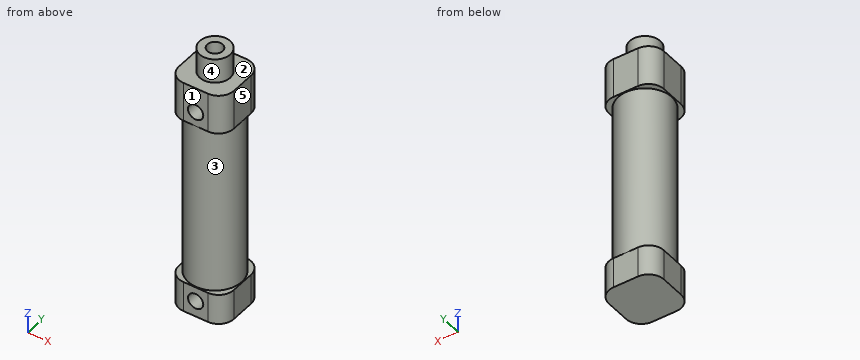
```python
from build123d import *

# Parameters (mm, degrees)
SKETCH_1_W          = 18
SKETCH_1_H          = 18
EXTRUDE_1_DEPTH     = 10
SKETCH_2_R          = 8.75
EXTRUDE_2_DEPTH     = 55.5
SKETCH_3_W          = 18
SKETCH_3_H          = 18
EXTRUDE_3_DEPTH     = 13
SKETCH_4_R          = 5
EXTRUDE_4_DEPTH     = 8
SKETCH_5_R          = 2.5
CUT_EXTRUDE_1_DEPTH = 85.5
FILLET_1_R          = 5
CUT_EXTRUDE_2_REACH = 20
SKETCH_6_R          = 2.5


with BuildPart() as part:
    # 草图1 → 凸台-拉伸1 (new body)
    with BuildSketch(Plane.XY):
        Rectangle(SKETCH_1_W, SKETCH_1_H)
    extrude(amount=EXTRUDE_1_DEPTH)

    # 草图2 → 凸台-拉伸2 (add)
    with BuildSketch(Plane.XY.offset(10)):
        Circle(SKETCH_2_R)
    extrude(amount=EXTRUDE_2_DEPTH)

    # 草图3 → 凸台-拉伸3 (add)
    with BuildSketch(Plane.XY.offset(65.5)):
        Rectangle(SKETCH_3_W, SKETCH_3_H)
    extrude(amount=EXTRUDE_3_DEPTH)

    # 草图4 → 凸台-拉伸4 (add)
    with BuildSketch(Plane.XY.offset(78.5)):
        Circle(SKETCH_4_R)
    extrude(amount=EXTRUDE_4_DEPTH)

    # 草图5 → 切除-拉伸1 (cut)
    with BuildSketch(Plane.XY.offset(86.5)):
        Circle(SKETCH_5_R)
    extrude(amount=-CUT_EXTRUDE_1_DEPTH, mode=Mode.SUBTRACT)

    # 圆角1
    fillet_1_edges = [part.edges().sort_by_distance(p)[0] for p in [
        (9, -9, 72),
        (9, 9, 72),
        (-9, 9, 72),
        (-9, -9, 72),
        (9, -9, 5),
        (-9, -9, 5),
        (-9, 9, 5),
        (9, 9, 5),
    ]]
    fillet(fillet_1_edges, radius=FILLET_1_R)

    # 草图6 → 切除-拉伸2 (cut, up to next)
    with BuildSketch(Plane.XZ.offset(9), mode=Mode.PRIVATE) as cut_extrude_2_sk1:
        with Locations((0, 5.25)):
            Circle(SKETCH_6_R)
    cut_extrude_2_tool1 = extrude(cut_extrude_2_sk1.sketch, amount=-CUT_EXTRUDE_2_REACH, mode=Mode.PRIVATE) & part.part
    add(cut_extrude_2_tool1.solids().sort_by_distance((0, -9, 5.25))[0], mode=Mode.SUBTRACT)
    # 草图6 → 切除-拉伸2 (cut, up to next)
    with BuildSketch(Plane.XZ.offset(9), mode=Mode.PRIVATE) as cut_extrude_2_sk2:
        with Locations((0, 70.25)):
            Circle(SKETCH_6_R)
    cut_extrude_2_tool2 = extrude(cut_extrude_2_sk2.sketch, amount=-CUT_EXTRUDE_2_REACH, mode=Mode.PRIVATE) & part.part
    add(cut_extrude_2_tool2.solids().sort_by_distance((0, -9, 70.25))[0], mode=Mode.SUBTRACT)


solid = part.part
```
Verification items for the finished model (mm, model axes). Face numbers are marked on the shaded views. A direction names the side the tool comes from. Round coordinates to 2 decimals unless told otherwise and drop trailing zeros. Order: outer loops, then holes, each group sorted by start corner. A loop starts at its lowest first (then second) coordinate and runs counter-clockwise, first axis right, second up.
1) Cross-section at C-C, the plane z = 76. Record the cut outline in (x, y), plus the area to 3 significant figures.
Geometry says:
outline: (-9, -4) arc R5 ccw to (-4, -9) - (4, -9) arc R5 ccw to (9, -4) - (9, 4) arc R5 ccw to (4, 9) - (-4, 9) arc R5 ccw to (-9, 4) - close; hole circle Ø5 at (0, 0)
area: 283 mm2
2) Draft check along Z on the marked faces 1, 2 and 3. Enter one of: +Z half, -Z half, draft (parallel to the pull), parting line (faces both ways), or undercut.
Geometry says:
face 1: draft
face 2: +Z half
face 3: undercut
3) Depth check by flat-ended pin: pin 1 (4 mm diameter, centred on x = -5.5, z = 26, fed in from -Y); pin 2 (6 mm diameter, centred on y = -6, z = 42.5, fed in from -X); pin 3 (1 mm diameter, centred on y = 6.5, z = 69.5, fed in from +X). Enter the tip coordinate at first touch or a pass-through.
Geometry says:
pin 1: stops at y = -8.02
pin 2: stops at x = -8.22
pin 3: stops at x = 8.58
4) Cross-section at B-B, the plane x = -7. Record the cut outline in (y, z), plus the area to 3 significant figures.
Geometry says:
outline: (-8, 0) - (8, 0) - (8, 10) - (5.25, 10) - (5.25, 65.5) - (8, 65.5) - (8, 78.5) - (-8, 78.5) - (-8, 65.5) - (-5.25, 65.5) - (-5.25, 10) - (-8, 10) - close
area: 951 mm2
5) Cross-section at D-D, the plane y = -6.5. Record the cut outline in (x, z).
Geometry says:
outline: (-8.33, 0) - (8.33, 0) - (8.33, 10) - (5.86, 10) - (5.86, 65.5) - (8.33, 65.5) - (8.33, 78.5) - (-8.33, 78.5) - (-8.33, 65.5) - (-5.86, 65.5) - (-5.86, 10) - (-8.33, 10) - close; hole circle Ø5 at (0, 5.25); hole circle Ø5 at (0, 70.25)
6) Material ranges on line 1 (Z direction, x = 0, y = -3.5); line 2 (Y direction, x = 0, z = 31.5); line 3 (Z direction, x = 0, y = -6.25), recorded low to high.
Geometry says:
line 1: z = 0 to 2.75, 7.75 to 67.75, 72.75 to 86.5
line 2: y = -8.75 to -2.5, 2.5 to 8.75
line 3: z = 0 to 2.75, 7.75 to 67.75, 72.75 to 78.5
7) Cross-section at A-A, the plane x = 0. Record the cut outline in (y, z), plus the area to 3 significant figures.
Geometry says:
outline: (-9, 0) - (9, 0) - (9, 10) - (8.75, 10) - (8.75, 65.5) - (9, 65.5) - (9, 78.5) - (5, 78.5) - (5, 86.5) - (2.5, 86.5) - (2.5, 1) - (-2.5, 1) - (-2.5, 2.75) - (-9, 2.75) - close; (-9, 7.75) - (-2.5, 7.75) - (-2.5, 67.75) - (-9, 67.75) - (-9, 65.5) - (-8.75, 65.5) - (-8.75, 10) - (-9, 10) - close; (-9, 72.75) - (-2.5, 72.75) - (-2.5, 86.5) - (-5, 86.5) - (-5, 78.5) - (-9, 78.5) - close
area: 973 mm2
8) Tool access check on the marked faces 4 and 5. Record the directions out of +Z, -Z, +X, -X, +Y, -Y that give a thin tool (end or side, any length) a straight path to the whole face; none if there is none.
Geometry says:
face 4: +Z
face 5: +Z, -Z, +X, +Y, -Y
